Can you work these out from the drawing? Everything is in mm from the part's minimum corner. A direction names the side the tool comes from. Coordinates: 2 decimals unless noted, no trailing zeros. Write each loop counter-clockwise with the first axis right and the second up, starting at its lowest first coordinate (ties: lowest second). Pieces come first, ordered by that corner, then holes. Notation, with made-up numbers: M 86.5,85.5 L 107.5,85.5 A23 ccw 107.5,120.5 Z; hole C 15.25,20 d7. An arc over 180 degrees is marked long. Answer as a JSON object with one key per item and string values. Group by question number.
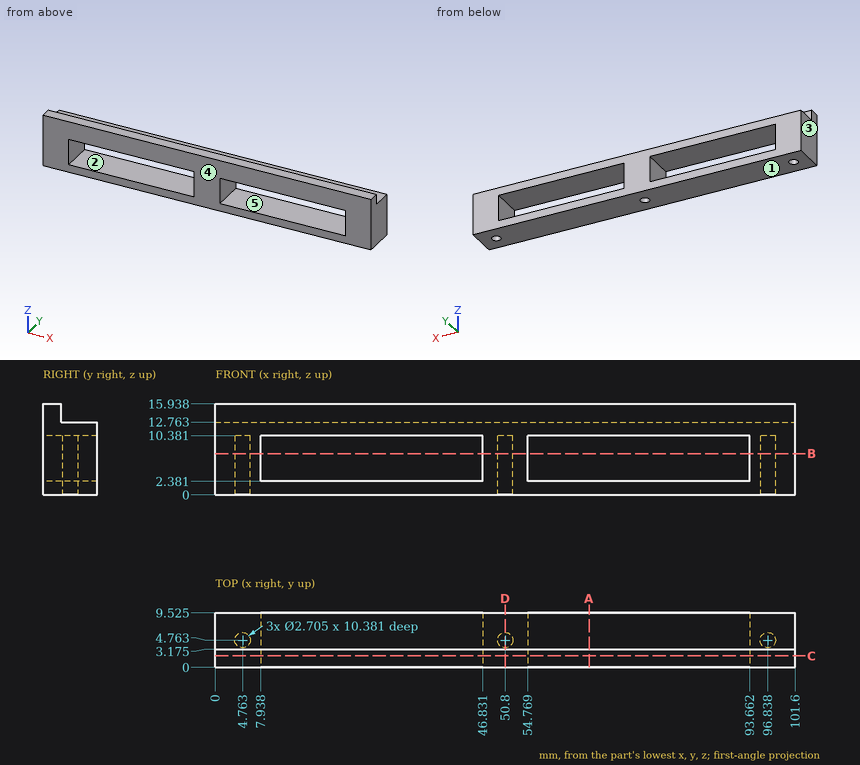
Q1. If we section it at D-D on x = 50.8: List the corners of the cut face in (y, z) for me (1 decimal).
Q2. If we section it at C-C on y = 2: List the corners of the cut face in (x, z) for me, and give its area (3 significant figures).
Q3. We'd pull the mould along Z, two halves only. Please class the marked faces 1, 2 and 3: pulls with the +Z half, pulls with the -Z half, needs draft (parallel to the pull), parting line crosses it, or undercut.
Q4. On a 3-axis mill with a long thin cutter (end or side, diameter ignored), from which of +Z, -Z, +X, -X, +Y, -Y can I reach the whole of each face in a straight line? I mean the marked faces 4 and 5. Say none if no direction works.
Q5. Will these pins go through, and if not, where does the flat tip stop? pin 1 (2.5 mm diameter, centred on x = 66, z = 14.5, fed in from +Y) (1 decimal); pin 2 (0.8 mm diameter, centred on x = 5, y = 5, fed in from -Z); pin 3 (2.5 mm diameter, centred on x = 50.8, y = 4.76, fed in from +Z).
Q6. Please list where these lines run through material, in increasing order: L1, parallel to X at y = 1.25, z = 2.5; L2, parallel to Z at x = 55, y = 4.25; L3, parallel to X at y = 4.5, z = 6.25 (1 decimal).
Q7. If we section it at A-A on x = 65.5: List the corners of the cut face in (y, z) for me (1 decimal).
Q8. If we section it at B-B on z = 7.25: List the corners of the cut face in (x, y) for me (1 decimal).
Reply:
{
 "1": {"outline": "M 0,0 L 3.4,0 L 3.4,10.4 L 6.1,10.4 L 6.1,0 L 9.5,0 L 9.5,12.8 L 3.2,12.8 L 3.2,15.9 L 0,15.9 Z"},
 "2": {"outline": "M 0,0 L 101.6,0 L 101.6,15.94 L 0,15.94 Z; hole M 7.94,2.38 L 46.83,2.38 L 46.83,10.38 L 7.94,10.38 Z; hole M 54.77,2.38 L 93.66,2.38 L 93.66,10.38 L 54.77,10.38 Z", "area": "997 mm^2"},
 "3": {"face 1": "pulls with the -Z half", "face 2": "undercut", "face 3": "needs draft"},
 "4": {"face 4": "+Z, -Z, +X, -X, -Y", "face 5": "+Y, -Y"},
 "5": {"pin 1": "y = 3.2", "pin 2": "z = 10.38", "pin 3": "z = 12.76"},
 "6": {"L1": "0 to 7.94, 46.83 to 54.77, 93.66 to 101.6", "L2": "0 to 2.38, 10.38 to 12.76", "L3": "0 to 3.4, 6.1 to 7.9, 46.8 to 49.5, 52.1 to 54.8, 93.7 to 95.5, 98.2 to 101.6"},
 "7": {"outline": "M 0,0 L 9.5,0 L 9.5,2.4 L 0,2.4 Z; M 0,10.4 L 9.5,10.4 L 9.5,12.8 L 3.2,12.8 L 3.2,15.9 L 0,15.9 Z"},
 "8": {"outline": "M 0,0 L 7.9,0 L 7.9,9.5 L 0,9.5 Z; M 46.8,0 L 54.8,0 L 54.8,9.5 L 46.8,9.5 Z; M 93.7,0 L 101.6,0 L 101.6,9.5 L 93.7,9.5 Z; hole C 4.8,4.8 d2.7; hole C 50.8,4.8 d2.7; hole C 96.8,4.8 d2.7"}
}
